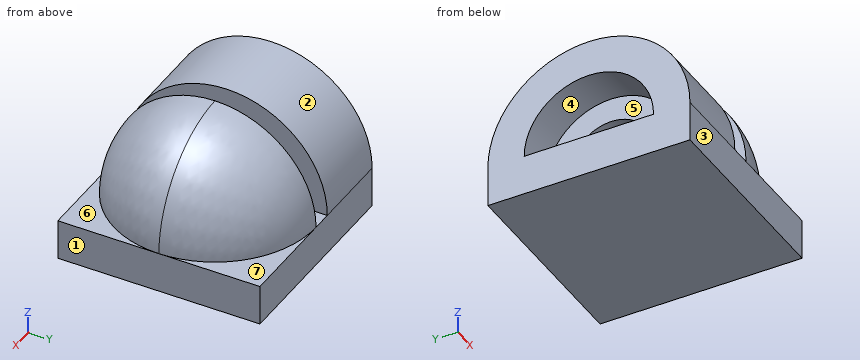
```python
from build123d import *

# Parameters (mm, degrees)
F0_W     = 25
F0_H     = 25
F1_DEPTH = 5
F3_ANGLE = 90
F5_DEPTH = 10
F6_DEPTH = 5


with BuildPart() as f1:
    # F0 (on Top) → F1 (new body)
    with BuildSketch(Plane.XY):
        Rectangle(F0_W, F0_H)
    extrude(amount=F1_DEPTH)

    # F2 (on face) → F3 (revolve)
    with BuildSketch(Plane.XY.offset(5)):
        with BuildLine():
            ThreePointArc((12.5, 0), (8.838835, 8.838835), (0, 12.5))
            Line((0, 12.5), (0, -12.5))
            ThreePointArc((0, -12.5), (8.838835, -8.838835), (12.5, 0))
        make_face()
    revolve(axis=Axis((0, 0, 5), (0, -1, 0)), revolution_arc=F3_ANGLE)

    # F4 (on face) → F5 (join)
    with BuildSketch(Plane(origin=(-12.5, 0, 0), x_dir=(0, -1, 0), z_dir=(-1, 0, 0))):
        with BuildLine():
            Line((8, 5), (12.5, 5))
            ThreePointArc((12.5, 5), (0, 17.5), (-12.5, 5))
            Line((-12.5, 5), (-8, 5))
            ThreePointArc((-8, 5), (0, 13), (8, 5))
        make_face()
        with BuildLine():
            Line((5, 5), (8, 5))
            ThreePointArc((8, 5), (0, 13), (-8, 5))
            Line((-8, 5), (-5, 5))
            ThreePointArc((-5, 5), (0, 10), (5, 5))
        make_face()
    extrude(amount=-F5_DEPTH)

    # F4 (on face) → F6 (cut)
    with BuildSketch(Plane(origin=(-12.5, 0, 0), x_dir=(0, -1, 0), z_dir=(-1, 0, 0))):
        with BuildLine():
            Line((5, 5), (8, 5))
            ThreePointArc((8, 5), (0, 13), (-8, 5))
            Line((-8, 5), (-5, 5))
            ThreePointArc((-5, 5), (0, 10), (5, 5))
        make_face()
    extrude(amount=-F6_DEPTH, mode=Mode.SUBTRACT)


solid = f1.part
```
Model file for the job. Use its own axes, mm. Face numbers are marked on the shaded views. A direction names the side the tool comes from. Coordinates: 2 decimals unless noted, no trailing zeros. Loops run counter-clockwise (first coordinate to the right, second up) from the corner with the lowest first, then second, coordinate; pieces in that order, holes last. Notation, with made-up numbers: (36, 24.5) - (85, 24.5) arc R31 ccw to (85, 50.5) - close; hole circle Ø10 at (48.25, -25.5). An arc over 180 degrees is marked (long way). Answer as a JSON object with one key per item and string values. Group by question number.
(1) Flat gauge pins, fed straight in: pin 1 (10 mm diameter, centred on y = -1, z = 6.5, fed in from -X); pin 2 (1 mm diameter, centred on x = -6, z = 10.5, fed in from +Y); pin 3 (4 mm diameter, centred on x = -1, z = 14.5, fed in from -Y); pin 4 (14 mm diameter, centred on x = 8, y = -7.5, fed in from +Z). Where does each tip first touch, or does it go through?
(2) Cut at A-A (x = -9.25). Give the cut face in (y, z), then the cut area to 3 significant figures.
(3) Probe line 1 along Z through (x, y) = (-4.75, -2.5); line 2 along Y through (x, z) = (-10, 6.5); line 3 along Z through (x, y) = (6.75, -9.25). List the from-to ranges inside material, lowest first.
(4) Two-plate mould, pull along Y, no slides. Class the marked faces 1, 2, 3 and 4: released by +Y, released by -Y, zero draft, split by the parting line, or undercut.
(5) Cut at B-B (z = 9). State how many separate pieces and enclosed holes the cut face has, then the cut area to 3 significant figures.
(6) Tool access for the marked faces 5, 6 and 7: list every direction of +Z, -Z, +X, -X, +Y, -Y with a clear straight run to the whole face (end or side of a thin tool).
Geometry says:
{
 "1": {"pin 1": "stops at x = -12.5", "pin 2": "stops at y = 11.46", "pin 3": "stops at y = -9.79", "pin 4": "stops at z = 16.85"},
 "2": {"outline": "(-12.5, 0) - (12.5, 0) - (12.5, 5) arc R12.5 ccw to (-12.5, 5) - close; hole (-8, 5) - (8, 5) arc R8 ccw to start", "area": "270 mm^2"},
 "3": {"line 1": "z = 0 to 5, 9.33 to 17.25", "line 2": "y = -12.41 to -7.86, 7.86 to 12.41", "line 3": "z = 0 to 10.01"},
 "4": {"face 1": "zero draft", "face 2": "split by the parting line", "face 3": "released by -Y", "face 4": "undercut"},
 "5": {"separate pieces": "3", "enclosed holes": "0", "area": "358 mm^2"},
 "6": {"face 5": "-X", "face 6": "+Z, +X, -Y", "face 7": "+Z, +X, +Y"}
}
